from build123d import *

# Parameters (mm, degrees)
F0_W     = 36
F0_H     = 1.5
F0_H_2   = 21.5
F1_DEPTH = 3
F2_DEPTH = 4
F3_D     = 3
F3_DEPTH = 8
F3_TIP   = 0.9012909285
F4_R     = 1
F6_DEPTH = 25
F8_DEPTH = 25


with BuildPart() as f1:
    # F0 (on Top) → F1 (new body)
    with BuildSketch(Plane.XY):
        with Locations((-1.819640398, 8.1819643453)):
            Rectangle(F0_W, F0_H)
        with Locations((-1.819640398, -3.3180356547)):
            Rectangle(F0_W, F0_H_2)
        with BuildLine():
            ThreePointArc((-17.819640398, 0.7696866851), (-13.8447666639, 1.4570906111), (-13.1573627379, 5.4319643453))
            Line((-13.1573627379, 5.4319643453), (14.180359602, 5.4319643453))
            Line((14.180359602, 5.4319643453), (14.180359602, -7.4057579946))
            ThreePointArc((14.180359602, -7.4057579946), (10.2054858678, -8.0931619206), (9.5180819418, -12.0680356547))
            Line((9.5180819418, -12.0680356547), (-17.819640398, -12.0680356547))
            Line((-17.819640398, -12.0680356547), (-17.819640398, 0.7696866851))
        make_face(mode=Mode.SUBTRACT)
        with Locations((-1.819640398, -14.8180356547)):
            Rectangle(F0_W, F0_H)
    extrude(amount=F1_DEPTH)

    # F0 (on Top) → F2 (join)
    with BuildSketch(Plane.XY):
        with Locations((-1.819640398, 8.1819643453)):
            Rectangle(F0_W, F0_H)
        with Locations((-1.819640398, -14.8180356547)):
            Rectangle(F0_W, F0_H)
    extrude(amount=F2_DEPTH)

    # F3
    with Locations(Plane(origin=(0, 0, 0), x_dir=(1, 0, 0), z_dir=(0, 0, -1))):
        with Locations((12.680359602, 10.5680356547), (-16.319640398, -3.9319643453)):
            Hole(F3_D / 2, depth=F3_DEPTH)
            with Locations((0, 0, -(F3_DEPTH + F3_TIP / 2))):  # 118° drill point
                Cone(0, F3_D / 2, F3_TIP, mode=Mode.SUBTRACT)

    # F4
    f4_edges = [f1.edges().sort_by_distance(p)[0] for p in [
        (-1.81964, 8.931964, 4),
        (-1.81964, -15.568036, 4),
    ]]
    fillet(f4_edges, radius=F4_R)

    # F5 (on face) → F6 (cut)
    with BuildSketch(Plane(origin=(-19.819640398, 0, 0), x_dir=(0, -1, 0), z_dir=(-1, 0, 0))):
        with BuildLine():
            Line((7.5680356547, 1.5), (4.5680356547, 1.5))
            ThreePointArc((4.5680356547, 1.5), (3.1191469153, -0.3882285677), (5.3180356547, -1.2990381057))
            ThreePointArc((5.3180356547, -1.2990381057), (6.0680356547, -1.5), (6.8180356547, -1.2990381057))
            ThreePointArc((6.8180356547, -1.2990381057), (9.0169243942, -0.3882285677), (7.5680356547, 1.5))
        make_face()
    extrude(amount=-F6_DEPTH, mode=Mode.SUBTRACT)

    # F7 (on face) → F8 (cut)
    with BuildSketch(Plane.YZ.offset(16.180359602)):
        with BuildLine():
            ThreePointArc((-0.5680356547, 0), (0.9319643453, -1.5), (2.4319643453, 0))
            ThreePointArc((2.4319643453, 0), (1.9926245171, 1.0606601718), (0.9319643453, 1.5))
            ThreePointArc((0.9319643453, 1.5), (-0.1286958265, 1.0606601718), (-0.5680356547, 0))
        make_face()
        with BuildLine():
            ThreePointArc((-0.5680356547, 0), (-0.1286958265, 1.0606601718), (0.9319643453, 1.5))
            Line((0.9319643453, 1.5), (-2.0680356547, 1.5))
            ThreePointArc((-2.0680356547, 1.5), (-1.0073754829, 1.0606601718), (-0.5680356547, 0))
        make_face()
        with BuildLine():
            ThreePointArc((-2.0680356547, 1.5), (-3.1286958265, -1.0606601718), (-0.5680356547, 0))
            ThreePointArc((-0.5680356547, 0), (-1.0073754829, 1.0606601718), (-2.0680356547, 1.5))
        make_face()
    extrude(amount=-F8_DEPTH, mode=Mode.SUBTRACT)


solid = f1.part
Model file for the job. Use its own axes, mm. A direction names the side the tool comes from. Coordinates: 2 decimals unless noted, no trailing zeros. Write each loop counter-clockwise with the first axis right and the second up, starting at its lowest first coordinate (ties: lowest second). Pieces come first, ordered by that corner, then holes. Notation, with made-up numbers: (2, -15.5) - (47, -15.5) arc R18 cw to (47, 18.5) - close; hole circle Ø7 at (72, -34.75). An arc over 180 degrees is marked (long way). Write each question's results on one line, items separated by ' | '. Start each with the question number.
1) 3-axis set-ups, long thin cutter, end or side, ignore diameter. For faces 1 (the face through (15, -1, 1.5)), 2 (the face through (-19, -6, 1.5)), 3 (the face through (-2.1, -14.068, 3.5)): which of +Z, -Z, +X, -X, +Y, -Y reach the whole face in a straight line?
2) Cut at C-C (x = -6). Write the cut outline in (y, z), then the cut area to 3 significant figures.
3) Mould opens along Y. For faces 4 (the face through (10.2, -8.1, 1.5)), 5 (the face through (-6, 6, 0)), 6 (the face through (-1.568, 8.647, 3.699)) say: pulls with the +Y half, pulls with the -Y half, needs draft (parallel to the pull), parting line crosses it, or undercut.
4) Flat gauge pins, fed straight in: P1, Ø2, axis at y = -7.5, z = 1, coming from the -X side; P2, Ø1.6, axis at x = 14.5, y = -0.5, coming from the -Z side; P3, Ø0.5, axis at x = -5, z = 3.5, coming from the -Y side; P4, Ø3.5, axis at x = 12.68, y = -10.57, coming from the +Z side. Where does each tip first touch, or does it go through?
5) Cut at B-B (z = 0.55). Write the cut outline in (x, y).
6) Probe line 1 along X through (y, z) = (4, 0.35); line 2 along Y through (x, z) = (-1, 0.65); line 3 along X through (y, z) = (-5.25, 2.7). List the from-to ranges inside material, lowest first. Write a range as from..to.
7) Cut at A-A (y = 0). Write the cut outline in (x, z), then the cut area to 3 significant figures.
8) Cut at D-D (z = 3.45). Write the cut outline in (x, y) (3 decimals), then the cut area to 3 significant figures.
Returned:
1) face 1: -Z, +X | face 2: -Z, -X | face 3: +Z, +X, -X
2) outline: (-15.57, 0) - (-12.07, 0) - (-12.07, 3) - (-14.07, 3) - (-14.07, 4) - (-14.57, 4) arc R1 ccw to (-15.57, 3) - close; (5.43, 0) - (8.93, 0) - (8.93, 3) arc R1 ccw to (7.93, 4) - (7.43, 4) - (7.43, 3) - (5.43, 3) - close | area: 23.6 mm^2
3) face 4: undercut | face 5: needs draft | face 6: pulls with the +Y half
4) P1: x = -19.82 | P2: z = 1.5 | P3: y = -15.54 | P4: z = 3
5) outline: (-19.82, -15.57) - (16.18, -15.57) - (16.18, -3.46) - (14.18, -3.46) - (14.18, -7.41) arc R3.5 ccw to (9.52, -12.07) - (-17.82, -12.07) - (-17.82, -8.96) - (-19.82, -8.96) - close; (-19.82, -3.17) - (-17.82, -3.17) - (-17.82, 0.77) arc R3.5 ccw to (-13.16, 5.43) - (14.18, 5.43) - (14.18, 2.33) - (16.18, 2.33) - (16.18, 8.93) - (-19.82, 8.93) - close; hole circle Ø3 at (-16.32, 3.93); hole circle Ø3 at (12.68, -10.57)
6) line 1: -19.82..-17.82, -14.82..-12.82, 14.18..16.18 | line 2: -15.57..-12.07, 5.43..8.93 | line 3: -19.82..-17.82, 14.18..16.18
7) outline: (-19.82, 0) - (-17.82, 0) - (-17.82, 3) - (-19.82, 3) - close; (14.18, 1.5) - (16.18, 1.5) - (16.18, 3) - (14.18, 3) - close | area: 9.00 mm^2
8) outline: (-19.82, -15.461) - (16.18, -15.461) - (16.18, -14.068) - (-19.82, -14.068) - close; (-19.82, 7.432) - (16.18, 7.432) - (16.18, 8.825) - (-19.82, 8.825) - close | area: 100 mm^2
